Geometry check sheet. Reference: the model listing, model coordinates, mm. Give positions to 0.01 mm unless a question says otherwise; leave off trailing zeros. Write each loop counter-clockwise with the first axis right and the second up, starting at its lowest first coordinate (ties: lowest second). Pieces come first, ordered by that corner, then holes. Notation, with made-up numbers: M 22.25,-5.75 L 75.25,-5.75 A15 ccw 75.25,17.25 Z; hole C 5.5,36 d1. An arc over 180 degrees is marked long. Use one line per item in the form item = value. Start each with the question number.
```python
from build123d import *

# Parameters (mm, degrees)
SKETCH2_R           = 37.5
BOSS_EXTRUDE1_DEPTH = 500
SKETCH3_R           = 35.7
CUT_EXTRUDE1_DEPTH  = 500
SKETCH4_W           = 100
SKETCH4_H           = 36
CUT_EXTRUDE2_DEPTH  = 500


with BuildPart() as part:
    # Sketch2 → Boss-Extrude1 (new body)
    with BuildSketch(Plane.XY):
        Circle(SKETCH2_R)
    extrude(amount=BOSS_EXTRUDE1_DEPTH)

    # Sketch3 → Cut-Extrude1 (cut)
    with BuildSketch(Plane.XY.offset(500)):
        Circle(SKETCH3_R)
    extrude(amount=-CUT_EXTRUDE1_DEPTH, mode=Mode.SUBTRACT)

    # Sketch4 → Cut-Extrude2 (cut, symmetric)
    with BuildSketch(Plane(origin=(0, 0, 0), x_dir=(0, 0, -1), z_dir=(1, 0, 0))):
        with Locations((-50, -0.380488828)):
            Rectangle(SKETCH4_W, SKETCH4_H)
    extrude(amount=CUT_EXTRUDE2_DEPTH, both=True, mode=Mode.SUBTRACT)


solid = part.part
```
(1) Sectioned sample at C-C, the plane z = 372.5. Record the boundary of the cut face in (x, y).
(2) Depth check by flat-ended pin: pin 1 (1 mm diameter, centred on x = -32.5, z = 50.5, fed in from -Y); pin 2 (2 mm diameter, centred on x = -33, y = -2, fed in from -Z); pin 3 (7.5 mm diameter, centred on x = 33, y = 2, fed in from -Z); pin 4 (1 mm diameter, centred on y = -28.5, z = 368.5, fed in from +X). Enter the tip coordinate at first touch or a pass-through.
(3) Draft check along Y on faces 1 (the cylindrical face through (-37.464, 1.649, 246.5)), 2 (the flat face through (0, 36, 0)), 3 (the cylindrical face through (-35.665, 1.57, 253.5)). Enter one of: released by +Y, released by -Y, zero draft, split by the parting line, or undercut.
(4) Sectioned sample at A-A, the plane x = 0. Record the boundary of the cut face in (y, z).
(5) Sectioned sample at B-B, the plane y = 0. Record the boundary of the cut face in (x, z), plus the area to 3 significant figures.
(6) Thickness scan on probe 1 along X at (y, z) = (0, 275.5); probe 2 along Z at (x, y) = (-33, 15.5). Record the ranges inside material, lowest first. Write a range as [from, to].
Numbers:
q1.outline = C 0,0 d75; hole C 0,0 d71.4
q2.pin_1 = -19.55
q2.pin_2 = through
q2.pin_3 = 100
q2.pin_4 = 24.94
q3.face_1 = split by the parting line
q3.face_2 = zero draft
q3.face_3 = undercut
q4.outline = M -37.5,0 L -35.7,0 L -35.7,500 L -37.5,500 Z; M 35.7,0 L 37.5,0 L 37.5,500 L 35.7,500 Z
q5.outline = M -37.5,100 L -35.7,100 L -35.7,500 L -37.5,500 Z; M 35.7,100 L 37.5,100 L 37.5,500 L 35.7,500 Z
q5.area = 1,440 mm2
q6.probe_1 = [-37.5, -35.7], [35.7, 37.5]
q6.probe_2 = [100, 500]
